Design review of the part built by this model. Coordinates are the model's own, in mm. A direction names the side the tool comes from. Coordinates: 2 decimals unless noted, no trailing zeros. Write each loop counter-clockwise with the first axis right and the second up, starting at its lowest first coordinate (ties: lowest second). Pieces come first, ordered by that corner, then holes.
Q1. Take a section at B-B (y = 39). Give the boundary of the cut face in (x, z).
Q2. Machinability: for faces 1 (the flat face through (0.2, 23.6, -20)), 2 (the flat face through (-21, 34, -25)), 3 (the flat face through (20, 34, -25)), 4 (the flat face through (35, 3, -5)), which of the approach directions +Z, -Z, +X, -X, +Y, -Y give a long, thin tool a straight path to every point of the face, cutting with its end or side? Answer none if there is none.
Q3. Take a section at D-D (x = 7). Give the boundary of the cut face in (y, z) (1 decimal).
Q4. Mouldability with a two-part tool opening along Z and no side actions: class faces 5 (the flat face through (46.6, 10, -18.5)), 6 (the cylindrical face through (60, 5, -25)), 7 (the cylindrical face through (-48.955, 4.93, -30.158)) as pulls with the +Z half, pulls with the -Z half, needs draft (parallel to the pull), parting line crosses it, or undercut.
Q5. Take a section at C-C (z = -45.5). Give the boundary of the cut face in (x, y).
Q6. For probe 1 along X at (y, z) = (3, -25); probe 2 along Y at (x, z) = (-51, -36); probe 3 along Y at (x, z) = (-5, -40), list the stretches that pass through material, from the lowest coordinate up.
Q7. Insertion check: pin 1 (1.8 mm diameter, centred on y = 2, z = -45, fed in from -X); pin 2 (4 mm diameter, centred on y = 31, z = -29, fed in from -X); pin 3 (2 mm diameter, centred on y = 42.5, z = -33.5, fed in from +X). Each pin has a flat end and moves straight along its axis. Give the tip position at first contact, or say it passes through.
Q8. Take a section at A-A (z = -25). Give the boundary of the cut face in (x, y).
```python
from build123d import *

# Parameters (mm, degrees)
EXTRUDE_1_DEPTH     = 50
SKETCH_3_R          = 20
SKETCH_3_R_2        = 16
CUT_EXTRUDE_1_DEPTH = 10
CUT_EXTRUDE_2_DEPTH = 70.864153899
EXTRUDE_START       = -30
SKETCH_4_R          = 16
SKETCH_4_R_2        = 10
EXTRUDE_2_DEPTH     = 30
CUT_EXTRUDE_START   = 43.165151137
CUT_EXTRUDE_3_DEPTH = 6.834848863
SKETCH_6_R          = 6.5
EXTRUDE_3_DEPTH     = 10


# Read off the part's stored shape, not the designer's step: 切除-拉伸3
with BuildPart() as part:
    # 草图1 → 凸台-拉伸1 (new body)
    with BuildSketch(Plane.XY):
        Polygon((-35, 6), (-25, 34), (25, 34), (35, 6), (35, 0), (-35, 0), align=None)
    extrude(amount=-EXTRUDE_1_DEPTH)

    # 草图3 → 切除-拉伸1 (cut)
    with BuildSketch(Plane.XY):
        with Locations((0, 34)):
            Circle(SKETCH_3_R)
        with Locations((0, 34)):
            Circle(SKETCH_3_R_2, mode=Mode.SUBTRACT)
    extrude(amount=-CUT_EXTRUDE_1_DEPTH, mode=Mode.SUBTRACT)

    # 草图3<2> → 切除-拉伸2 (cut, through all)
    with BuildSketch(Plane.XY):
        with BuildLine():
            Line((-16, 34), (16, 34))
            ThreePointArc((16, 34), (0, 50), (-16, 34))
        make_face()
        with BuildLine():
            ThreePointArc((-16, 34), (0, 18), (16, 34))
            Line((16, 34), (-16, 34))
        make_face()
    extrude(amount=-CUT_EXTRUDE_2_DEPTH, mode=Mode.SUBTRACT)

    # 草图4 → 凸台-拉伸2 (add)
    with BuildSketch(Plane(origin=(0, 0, -50), x_dir=(-1, 0, 0), z_dir=(0, 0, -1)).offset(EXTRUDE_START)):
        with Locations((0, 34)):
            Circle(SKETCH_4_R)
        with Locations((0, 34)):
            Circle(SKETCH_4_R_2, mode=Mode.SUBTRACT)
    extrude(amount=EXTRUDE_2_DEPTH)

    # 切除-拉伸3 outline → 切除-拉伸3 (cut)
    with BuildSketch(Plane(origin=(0, 0, 0), x_dir=(1, 0, 0), z_dir=(0, 1, 0)).offset(CUT_EXTRUDE_START)):
        with BuildLine():
            add(Edge.make_bspline(
                [(3.99999996, 35), (3.999967414, 36.053927104), (3.563514164, 37.092301246), (2.830425635, 37.826427201), (2.096738851, 38.561151707), (1.06888327, 39), (-1.068884266, 39), (-2.100127628, 38.557285469), (-2.829510993, 37.827342841), (-3.558894179, 37.09740029), (-3.998804852, 36.060507963), (-4.001190045, 33.948526829), (-3.561222969, 32.904953883), (-2.829556469, 32.172702671), (-2.097890055, 31.440451664), (-1.056916053, 31.001093572), (1.048622532, 30.998910725), (2.090006878, 31.433217451), (2.82830312, 32.171448876), (3.566599135, 32.909680204), (3.999318272, 33.942605173), (3.999999722, 34.998278644), (3.999999987, 34.999139327), (3.99999996, 35)],
                knots=[0.750101996, 0.750101996, 0.750101996, 0.750101996, 0.875, 0.875, 0.875000116, 1, 1, 1.124999999, 1.124999999, 1.125000021, 1.249999998, 1.249999998, 1.374999984, 1.374999984, 1.375000009, 1.499999969, 1.499999969, 1.624999954, 1.624999954, 1.624999981, 1.749999938, 1.749999938, 1.750101934, 1.750101934, 1.750101934, 1.750101934], degree=3))
        make_face()
    extrude(amount=CUT_EXTRUDE_3_DEPTH, mode=Mode.SUBTRACT)

    # 草图6 → 凸台-拉伸3 (add)
    # profile 1 of 2: a face of its own
    with BuildSketch(Plane(origin=(0, 0, 0), x_dir=(1, 0, 0), z_dir=(0, 1, 0))):
        with BuildLine():
            Line((-35, 40), (-45, 40))
            ThreePointArc((-45, 40), (-60, 25), (-45, 10))
            Line((-45, 10), (-35, 10))
            Line((-35, 10), (35, 10))
            Line((35, 10), (35, 40))
            Line((35, 40), (-35, 40))
        make_face()
        with Locations(Location((-45, 25, 0), (0, 0, 270))):
            Circle(SKETCH_6_R, mode=Mode.SUBTRACT)
    # profile 2 of 2: a face of its own
    with BuildSketch(Plane(origin=(0, 0, 0), x_dir=(1, 0, 0), z_dir=(0, 1, 0))):
        with BuildLine():
            ThreePointArc((45, 40), (60, 25), (45, 10))
            Line((45, 10), (35, 10))
            Line((35, 10), (35, 40))
            Line((35, 40), (45, 40))
        make_face()
        with Locations(Location((45, 25, 0), (0, 0, 270))):
            Circle(SKETCH_6_R, mode=Mode.SUBTRACT)
    extrude(amount=EXTRUDE_3_DEPTH)


solid = part.part
```
Response:
1. outline: (-15.2, -50) - (-8.66, -50) - (-8.66, -20) - (-15.2, -20) - close; (8.66, -50) - (15.2, -50) - (15.2, -20) - (8.66, -20) - close
2. face 1: +Z, +Y
2. face 2: +Z, -Z, -X, +Y
2. face 3: +Z, -Z, +X, +Y
2. face 4: +Z, +X, +Y, -Y
3. outline: (0, -50) - (26.9, -50) - (26.9, -20) - (19.6, -20) - (19.6, -10) - (15.3, -10) - (15.3, 0) - (0, 0) - close; (41.1, -50) - (48.4, -50) - (48.4, -20) - (41.1, -20) - close
4. face 5: needs draft
4. face 6: parting line crosses it
4. face 7: undercut
5. outline: (-35, 0) - (35, 0) - (35, 6) - (25, 34) - (16, 34) arc R16 ccw to (-16, 34) - (-25, 34) - (-35, 6) - close; hole circle Ø20 at (0, 34)
6. probe 1: x = -60 to -51.5, -38.5 to 38.5, 51.5 to 60
6. probe 2: y = 0 to 10
6. probe 3: y = 0 to 25.34, 42.66 to 49.2
7. pin 1: stops at x = -35
7. pin 2: stops at x = -26.79
7. pin 3: stops at x = 14.13
8. outline: (-60, 0) - (-51.5, 0) - (-51.5, 10) - (-60, 10) - close; (-38.5, 0) - (38.5, 0) - (38.5, 10) - (33.57, 10) - (25, 34) - (16, 34) arc R16 ccw to (-16, 34) - (-25, 34) - (-33.57, 10) - (-38.5, 10) - close; (51.5, 0) - (60, 0) - (60, 10) - (51.5, 10) - close; hole circle Ø20 at (0, 34)
